Autodesk Inventor part; units mm, degrees
ref_plane "YZ Plane" through (0, 0, 0) normal (1, 0, 0) x (0, 1, 0)
ref_plane "XZ Plane" through (0, 0, 0) normal (0, 1, 0) x (-1, 0, 0)
ref_plane "XY Plane" through (0, 0, 0) normal (0, 0, 1) x (1, 0, 0)
sketch "Sketch1" plane through (0, 0, 0) normal (0, 0, 1) x (1, 0, 0)
  arc A0 (25.4, 0) -> (-25.4, 0) centre (0, 0) ccw
  line L0 (-25.4, 0) -> (-25.4, -19.05)
  line L1 (-25.4, -19.05) -> (-44.45, -19.05)
  line L2 (-44.45, -19.05) -> (-44.45, 19.05)
  line L3 (-44.45, 19.05) -> (-22.225, 38.1)
  line L4 (-22.225, 38.1) -> (-22.225, 69.85)
  line L5 (-22.225, 69.85) -> (-9.525, 69.85)
  line L6 (-9.525, 69.85) -> (-9.525, 38.1)
  line L7 (-9.525, 38.1) -> (0, 38.1)
  line L8 (0, 38.1) -> (0, -30.0357)
  line L9 (25.4, 0) -> (25.4, -19.05)
  line L10 (25.4, -19.05) -> (44.45, -19.05)
  line L11 (44.45, -19.05) -> (44.45, 19.05)
  line L12 (44.45, 19.05) -> (22.225, 38.1)
  line L13 (22.225, 38.1) -> (22.225, 69.85)
  line L14 (9.525, 69.85) -> (9.525, 38.1)
  line L15 (22.225, 69.85) -> (9.525, 69.85)
  line L16 (9.525, 38.1) -> (0, 38.1)
  dimension "d0" = 88.9
  dimension "d1" = 19.05
  dimension "d2" = 38.1
  dimension "d3" = 31.75
  dimension "d4" = 19.05
  dimension "d5" = 25.4
  dimension "d6" = 88.9
  dimension "d7" = 19.05
  dimension "d8" = 44.45
extrude "Extrusion1" add sketch "Sketch1" against normal blind 127
sketch "Sketch3" plane through (44.45, -19.05, 0) normal (1, 0, 0) x (0, 0, -1)
  line L0 (0, 88.9) -> (127, 88.9)
  line L1 (25.4, 88.9) -> (101.6, 88.9)
  line L2 (101.6, 88.9) -> (101.6, 76.2)
  line L3 (101.6, 76.2) -> (25.4, 76.2)
  line L4 (25.4, 76.2) -> (25.4, 88.9)
  line L5 (127, 88.9) -> (127, 57.15)
  line L6 (0, 57.15) -> (0, 88.9)
  line L7 (0, 0) -> (127, 0)
  line L8 (0, 57.15) -> (127, 57.15)
  line L9 (19.05, 0) -> (107.95, 0)
  line L10 (107.95, 0) -> (107.95, 57.15)
  line L11 (107.95, 57.15) -> (19.05, 57.15)
  line L12 (19.05, 57.15) -> (19.05, 0)
  line L13 (127, 38.1) -> (127, 0)
  line L14 (0, 0) -> (0, 38.1)
  point P0 (0, 19.05)
  point P1 (101.6, 82.55)
  point P2 (107.95, 0)
  dimension "d12" = 25.4
  dimension "d13" = 25.4
  dimension "d14" = 12.7
  dimension "d15" = 19.05
  dimension "d16" = 19.05
extrude "Extrusion2" cut sketch "Sketch3" against normal through all contours L0 L2 L3 L4 | L8 L10 L7 L12
sketch "Sketch4" plane through (22.225, 38.1, 0) normal (1, 0, 0) x (0, 0, -1)
  line L0 (0, 31.75) -> (25.4, 31.75)
  arc A0 (25.4, 31.75) -> (0, 31.75) centre (12.7, 31.75) ccw
  point P0 (0, -38.1)
extrude "Extrusion3" add sketch "Sketch4" against normal up to surface (12.7 mm away)
mirror "Mirror1" about plane through (0, 0, 0) normal (1, 0, 0) of "Extrusion3"
sketch "Sketch5" plane through (22.225, 38.1, -127) normal (1, 0, 0) x (0, 0, -1)
  arc A0 (-101.6, 31.75) -> (-127, 31.75) centre (-114.3, 31.75) ccw
  point P0 (-127, -38.1)
hole "Hole1" at (22.225, 69.85, -12.7) direction (-1, 0, 0) diameter 12.7 end through all
properties part number "TransferFork" material "Iron, Cast"
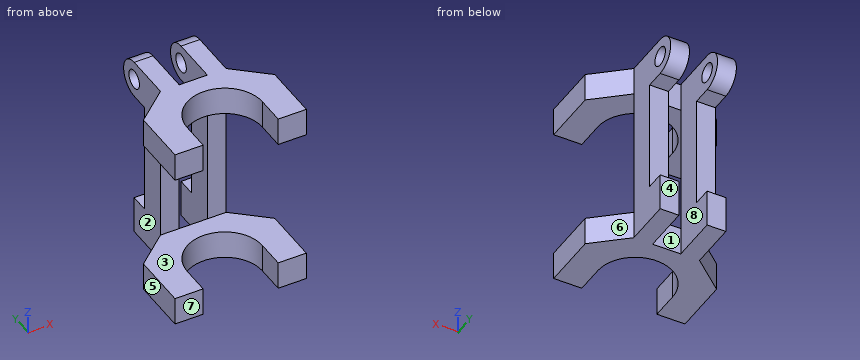
Verification items for the finished model (mm, model axes). Face numbers are marked on the shaded views. A direction names the side the tool comes from. Round coordinates to 2 decimals unless told otherwise and drop trailing zeros. Write each loop counter-clockwise with the first axis right and the second up, starting at its lowest first coordinate (ties: lowest second). Pieces come first, ordered by that corner, then holes. Notation, with made-up numbers: (39, 21) -> (74, 21) arc R20 cw to (74, 56) -> close; hole circle Ø5 at (27.25, 33.5). An arc over 180 degrees is marked (long way). Write each question's results on one line, items separated by ' | '.
Q1. Sectioned sample at A-A, the plane z = -104. Record the boundary of the cut face in (x, y) (3 decimals).
Derived:
outline: (-22.225, 38.1) -> (-9.525, 38.1) -> (-9.525, 69.85) -> (-22.225, 69.85) -> close; (9.525, 38.1) -> (22.225, 38.1) -> (22.225, 69.85) -> (9.525, 69.85) -> close
Q2. Access from +Z, -Z, +X, -X, +Y, -Y to the whole of each face (thin tool, end or side, straight path). Record for the marked faces 1, 2, 3, 4 and 5.
Derived:
face 1: +Z, -Z, +Y | face 2: +Z, -Z, -X, +Y | face 3: +X, -X, -Y | face 4: -Z, +X, -X, +Y | face 5: +Z, -Z, -X, +Y, -Y
Q3. Sectioned sample at C-C, the plane x = 0. Record the boundary of the cut face in (y, z), and give its area (3 significant figures).
Derived:
outline: (25.4, -127) -> (38.1, -127) -> (38.1, -107.95) -> (25.4, -107.95) -> close; (25.4, -19.05) -> (38.1, -19.05) -> (38.1, 0) -> (25.4, 0) -> close | area: 484 mm²
Q4. Thickness scan on probe 1 along X at (y, z) = (51, -117) (3 decimals); probe 2 along Z at (x, y) = (-13, 69); probe 3 along Z at (x, y) = (39, 16). Record the ranges inside material, lowest first.
Derived:
probe 1: x = -22.225 to -9.525, 9.525 to 22.225 | probe 2: z = -127 to -101.6, -25.4 to -18.99, -6.41 to 0 | probe 3: z = -127 to -107.95, -19.05 to 0
Q5. Go/stop test with flat-tipped pins: pin 1 Ø8 at (x, z) = (23.5, -66.5) entering from -Y; pin 2 Ø4 at (x, z) = (13.5, -64.5) entering from +Y; pin 3 Ø22 at (y, z) = (66.5, -52.5) entering from +X (3 decimals); pin 4 Ø10 at (x, y) = (27.5, 32.5) entering from +Z. Record where each tip stops, or that it passes through.
Derived:
pin 1: stops at y = 38.1 | pin 2: stops at y = 57.15 | pin 3: stops at x = 22.225 | pin 4: stops at z = 0
Q6. Sectioned sample at D-D, the plane z = -12.7. Record the boundary of the cut face in (x, y) (3 decimals), and give its area (3 significant figures).
Derived:
outline: (-44.45, -19.05) -> (-25.4, -19.05) -> (-25.4, 0) arc R25.4 cw to (25.4, 0) -> (25.4, -19.05) -> (44.45, -19.05) -> (44.45, 19.05) -> (22.225, 38.1) -> (22.225, 63.5) -> (9.525, 63.5) -> (9.525, 38.1) -> (-9.525, 38.1) -> (-9.525, 63.5) -> (-22.225, 63.5) -> (-22.225, 38.1) -> (-44.45, 19.05) -> close; (-22.225, 76.2) -> (-9.525, 76.2) -> (-9.525, 82.55) -> (-22.225, 82.55) -> close; (9.525, 76.2) -> (22.225, 76.2) -> (22.225, 82.55) -> (9.525, 82.55) -> close | area: 3,480 mm²
Q7. Draft check along X on the marked faces 6, 7 and 8. Enter one of: released by +X, released by -X, zero draft, split by the parting line, or undercut.
Derived:
face 6: released by +X | face 7: zero draft | face 8: undercut
Q8. Sectioned sample at B-B, the plane y = -6.5. Record the boundary of the cut face in (x, z).
Derived:
outline: (-44.45, -127) -> (-25.4, -127) -> (-25.4, -107.95) -> (-44.45, -107.95) -> close; (-44.45, -19.05) -> (-25.4, -19.05) -> (-25.4, 0) -> (-44.45, 0) -> close; (25.4, -127) -> (44.45, -127) -> (44.45, -107.95) -> (25.4, -107.95) -> close; (25.4, -19.05) -> (44.45, -19.05) -> (44.45, 0) -> (25.4, 0) -> close
